Verification items for the finished model (mm, model axes). A direction names the side the tool comes from. Round coordinates to 2 decimals unless told otherwise and drop trailing zeros. Loops run counter-clockwise (first coordinate to the right, second up) from the corner with the lowest first, then second, coordinate; pieces in that order, holes last. Notation, with made-up numbers: (8.25, 69.25) -> (31.25, 69.25) arc R21 ccw to (31.25, 79.25) -> close; hole circle Ø8 at (-20, 76). An arc over 180 degrees is marked (long way). Use a Markdown table: item, result. Add a question column.
```python
from build123d import *

# Parameters (mm, degrees)
BOSS_EXTRUDE1_DEPTH                             = 5
M5_CLEARANCE_HOLE1_D                            = 5.5
M5_CLEARANCE_HOLE1_DEPTH                        = 5
CSK_FOR_M3_FLAT_HEAD_MACHINE_SCREW1_D           = 3.4
CSK_FOR_M3_FLAT_HEAD_MACHINE_SCREW1_DEPTH       = 5
CSK_FOR_M3_FLAT_HEAD_MACHINE_SCREW1_CSINK_D     = 6.3
CSK_FOR_M3_FLAT_HEAD_MACHINE_SCREW1_CSINK_ANGLE = 90


with BuildPart() as part:
    # Sketch1 → Boss-Extrude1 (new body)
    with BuildSketch(Plane.XY):
        with BuildLine():
            Line((42, 0), (-42, 0))
            ThreePointArc((-42, 0), (-47.656854249, 2.343145751), (-50, 8))
            Line((-50, 8), (-50, 12))
            ThreePointArc((-50, 12), (-47.656854249, 17.656854249), (-42, 20))
            Line((-42, 20), (-25, 20))
            ThreePointArc((-25, 20), (-21.464466094, 21.464466094), (-20, 25))
            Line((-20, 25), (-20, 30))
            ThreePointArc((-20, 30), (-18.535533906, 33.535533906), (-15, 35))
            Line((-15, 35), (15, 35))
            ThreePointArc((15, 35), (18.535533906, 33.535533906), (20, 30))
            Line((20, 30), (20, 25))
            ThreePointArc((20, 25), (21.464466094, 21.464466094), (25, 20))
            Line((25, 20), (42, 20))
            ThreePointArc((42, 20), (47.656854249, 17.656854249), (50, 12))
            Line((50, 12), (50, 8))
            ThreePointArc((50, 8), (47.656854249, 2.343145751), (42, 0))
        make_face()
    extrude(amount=BOSS_EXTRUDE1_DEPTH)

    # M5 Clearance Hole1
    with Locations(Plane.XY.offset(5)):
        with Locations((-40, 10), (-25, 10), (25.25, 10), (40.125, 10)):
            Hole(M5_CLEARANCE_HOLE1_D / 2, depth=M5_CLEARANCE_HOLE1_DEPTH)

    # CSK for M3 Flat Head Machine Screw1
    with Locations(Plane(origin=(0, 0, 0), x_dir=(-1, 0, 0), z_dir=(0, 0, -1))):
        with Locations((-10, 17.5), (0, 7.5), (10, 17.5), (0, 27.5)):
            CounterSinkHole(CSK_FOR_M3_FLAT_HEAD_MACHINE_SCREW1_D / 2, CSK_FOR_M3_FLAT_HEAD_MACHINE_SCREW1_CSINK_D / 2, depth=CSK_FOR_M3_FLAT_HEAD_MACHINE_SCREW1_DEPTH, counter_sink_angle=CSK_FOR_M3_FLAT_HEAD_MACHINE_SCREW1_CSINK_ANGLE)


solid = part.part
```
1) Access from +Z, -Z, +X, -X, +Y, -Y to the whole of each face (thin tool, end or side, straight path). Record for faces 1 (the face through (9.779, 19.186, 3.25)), 2 (the face through (-20, 27, 2)).
2) Go/stop test with flat-tipped pins: pin 1 (2 mm diameter, centred on y = 25.5, z = 3.5, fed in from -X); pin 2 (2.5 mm diameter, centred on y = 27, z = 1.5, fed in from +X); pin 3 (4.5 mm diameter, centred on x = 10, y = 17.5, fed in from -Z). Record where each tip stops, or that it passes through.
3) Sectioned sample at D-D on x = 10. Enter the section's corners in (y, z).
4) Sectioned sample at A-A on x = -40. Enter the section's corners in (y, z).
5) Sectioned sample at B-B on z = 4.1. State how many separate pieces and enclosed holes the cut face has, then the cut area to 3 significant figures.
6) Thickness scan on line 1 (X direction, y = 17.5, z = 4.1); line 2 (X direction, y = 27.5, z = 2.75); line 3 (Y direction, x = -40, z = 3.5). Record the ranges inside material, lowest first.
7) Sectioned sample at C-C on y = 17.5. Enter the section's corners in (x, z).
8) Release check for a two-part mould opening along X. For faces 3 (the face through (47.719, 2.406, 2.465)), 4 (the face through (1, 14, 0)), 5 (the face through (-9.086, 18.933, 3.25)), 6 (the face through (-19, 33, 2)) record: released by +X, released by -X, zero draft, split by the parting line, or undercut.
Geometry results:
| question | item | result |
|---|---|---|
| 1 | face 1 | +Z, -Z |
| 1 | face 2 | +Z, -Z, -X, +Y |
| 2 | pin 1 | x = -20.03 |
| 2 | pin 2 | x = 20 |
| 2 | pin 3 | z = 0.9 |
| 3 | outline | (0, 0) -> (14.35, 0) -> (15.8, 1.45) -> (15.8, 5) -> (0, 5) -> close; (19.2, 1.45) -> (20.65, 0) -> (35, 0) -> (35, 5) -> (19.2, 5) -> close |
| 4 | outline | (0, 0) -> (7.25, 0) -> (7.25, 5) -> (0, 5) -> close; (12.75, 0) -> (20, 0) -> (20, 5) -> (12.75, 5) -> close |
| 5 | separate pieces | 1 |
| 5 | enclosed holes | 8 |
| 5 | area | 2,410 mm^2 |
| 6 | line 1 | -47.81 to -11.7, -8.3 to 8.3, 11.7 to 47.81 |
| 6 | line 2 | -20 to -1.7, 1.7 to 20 |
| 6 | line 3 | 0 to 7.25, 12.75 to 20 |
| 7 | outline | (-47.81, 0) -> (-13.15, 0) -> (-11.7, 1.45) -> (-11.7, 5) -> (-47.81, 5) -> close; (-8.3, 1.45) -> (-6.85, 0) -> (6.85, 0) -> (8.3, 1.45) -> (8.3, 5) -> (-8.3, 5) -> close; (11.7, 1.45) -> (13.15, 0) -> (47.81, 0) -> (47.81, 5) -> (11.7, 5) -> close |
| 8 | face 3 | released by +X |
| 8 | face 4 | zero draft |
| 8 | face 5 | undercut |
| 8 | face 6 | released by -X |
